The model under review builds one solid part; all positions refer to its coordinate system, in mm. Coordinates: 2 decimals unless noted, no trailing zeros. Order: outer loops, then holes, each group sorted by start corner. A loop starts at its lowest first (then second) coordinate and runs counter-clockwise, first axis right, second up. Notation, with made-up numbers: M -24,-21 L 19,-21 A15 cw 19,0 Z; hole C 61.25,49.5 d8. An arc over 180 degrees is marked long. Answer in a Markdown table with one row per item.
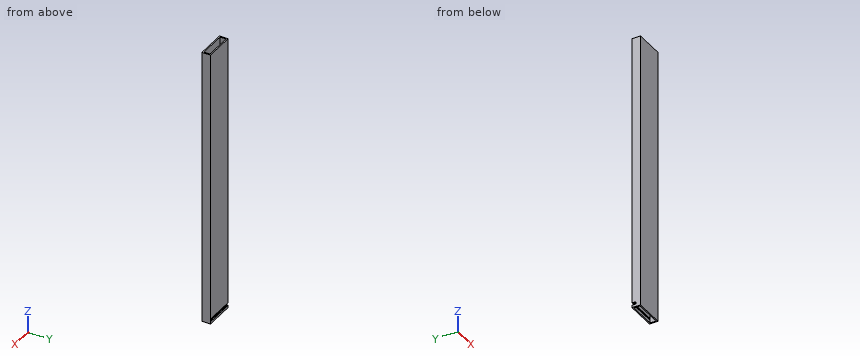
from build123d import *

# Parameters (mm, degrees)
SCHIZZO1_W                   = 35.931818182
SCHIZZO1_H                   = 10.2
SCHIZZO1_W_2                 = 33
SCHIZZO1_H_2                 = 7.2
ESTRUSIONE_ESTRUSIONE1_DEPTH = 330
SCHIZZO3_W                   = 2.7
SCHIZZO3_H                   = 3.2
TAGLIO_ESTRUSIONE1_DEPTH     = 34.465909091
TAGLIO_ESTRUSIONE2_DEPTH     = 1.5
SMUSSO2_SIZE                 = 0.6


with BuildPart() as part:
    # Schizzo1 → Estrusione-Estrusione1 (new body)
    with BuildSketch(Plane.XY):
        Rectangle(SCHIZZO1_W, SCHIZZO1_H)
        Rectangle(SCHIZZO1_W_2, SCHIZZO1_H_2, mode=Mode.SUBTRACT)
    extrude(amount=ESTRUSIONE_ESTRUSIONE1_DEPTH)

    # Schizzo3 → Taglio-Estrusione1 (cut)
    with BuildSketch(Plane.ZY.offset(17.965909091)):
        with Locations((4.35, 2)):
            Rectangle(SCHIZZO3_W, SCHIZZO3_H)
    extrude(amount=-TAGLIO_ESTRUSIONE1_DEPTH, mode=Mode.SUBTRACT)

    # Schizzo4 → Taglio-Estrusione2 (cut)
    with BuildSketch(Plane(origin=(0, 5.1, 0), x_dir=(1, 0, 0), z_dir=(0, 1, 0))):
        with BuildLine():
            Line((-16.5, -5.45), (15.4, -5.45))
            ThreePointArc((15.4, -5.45), (16.5, -4.35), (15.4, -3.25))
            Line((15.4, -3.25), (-16.5, -3.25))
            Line((-16.5, -3.25), (-16.5, -3))
            Line((-16.5, -3), (-17.965909091, -3))
            Line((-17.965909091, -3), (-17.965909091, -5.7))
            Line((-17.965909091, -5.7), (-16.5, -5.7))
            Line((-16.5, -5.7), (-16.5, -5.45))
        make_face()
    extrude(amount=-TAGLIO_ESTRUSIONE2_DEPTH, mode=Mode.SUBTRACT)

    # Smusso2
    smusso2_edges = [part.edges().sort_by_distance(p)[0] for p in [
        (-0.55, 5.1, 3.25),
        (16.5, 5.1, 4.35),
        (-0.55, 5.1, 5.45),
    ]]
    chamfer(smusso2_edges, length=SMUSSO2_SIZE)


solid = part.part
(1) Insertion check: P1, Ø1.6, axis at x = -17, z = 4.5, coming from the +Y side. The pin has a flat end and moves straight along its axis. Give the tip position at first contact, or say it passes through.
Report:
| item | result |
|---|---|
| P1 | y = 0.4 |
(2) To check wall thickness, follow line 1 (Y direction, x = -6, z = 68.5); line 2 (X direction, y = 2.25, z = 166); line 3 (Z direction, x = -7.5, y = 4.75). State the ranges of each line that lie inside material, in increasing order. Write a range as [from, to].
Report:
| item | result |
|---|---|
| line 1 | [-5.1, -3.6], [3.6, 5.1] |
| line 2 | [-17.97, -16.5], [16.5, 17.97] |
| line 3 | [0, 3], [5.7, 330] |
(3) Take a section at A-A (x = 2.5). Write out the cut boundary in (y, z), then the cut area to 3 significant figures.
Report:
| item | result |
|---|---|
| outline | M -5.1,0 L -3.6,0 L -3.6,330 L -5.1,330 Z; M 3.6,0 L 5.1,0 L 5.1,2.65 L 4.5,3.25 L 3.6,3.25 Z; M 3.6,5.45 L 4.5,5.45 L 5.1,6.05 L 5.1,330 L 3.6,330 Z |
| area | 986 mm^2 |
(4) Take a section at B-B (z = 51). Write out the cut boundary in (x, y).
Report:
| item | result |
|---|---|
| outline | M -17.97,-5.1 L 17.97,-5.1 L 17.97,5.1 L -17.97,5.1 Z; hole M -16.5,-3.6 L 16.5,-3.6 L 16.5,3.6 L -16.5,3.6 Z |
